from build123d import *

# Parameters (mm, degrees)
EXTRUDE_1_DEPTH          = 35
CUT_EXTRUDE_1_DEPTH      = 30
SKETCH_3_R               = 10
CUT_EXTRUDE_2_DEPTH      = 1
CUT_EXTRUDE_2_DEPTH_BACK = 71
CUT_EXTRUDE_3_DEPTH      = 5
HOLE_WIZARD_M4_1_D       = 3.3
HOLE_WIZARD_M4_1_DEPTH   = 5
HOLE_WIZARD_M4_2_D       = 3.3
HOLE_WIZARD_M4_2_DEPTH   = 5


with BuildPart() as part:
    # 스케치1 → 보스-돌출1 (new body)
    with BuildSketch(Plane(origin=(0, 0, 0), x_dir=(1, 0, 0), z_dir=(0, 1, 0))):
        with BuildLine():
            Line((-26, 35), (26, 35))
            ThreePointArc((26, 35), (61, 0), (26, -35))
            Line((26, -35), (-26, -35))
            ThreePointArc((-26, -35), (-61, 0), (-26, 35))
        make_face()
    extrude(amount=EXTRUDE_1_DEPTH)

    # 스케치2 → 컷-돌출1 (cut)
    with BuildSketch(Plane(origin=(0, 35, 0), x_dir=(1, 0, 0), z_dir=(0, 1, 0))):
        with BuildLine():
            Line((26, 30), (-26, 30))
            ThreePointArc((-26, 30), (-56, 0), (-26, -30))
            Line((-26, -30), (26, -30))
            ThreePointArc((26, -30), (56, 0), (26, 30))
        make_face()
    extrude(amount=-CUT_EXTRUDE_1_DEPTH, mode=Mode.SUBTRACT)

    # 스케치3 → 컷-돌출2 (cut, two sides)
    with BuildSketch(Plane.XY.offset(35)) as cut_extrude_2_sk:
        with Locations((0, 35)):
            Circle(SKETCH_3_R)
    extrude(amount=CUT_EXTRUDE_2_DEPTH, mode=Mode.SUBTRACT)
    extrude(cut_extrude_2_sk.sketch, amount=-CUT_EXTRUDE_2_DEPTH_BACK, mode=Mode.SUBTRACT)

    # 스케치4 → 컷-돌출3 (cut)
    with BuildSketch(Plane(origin=(0, 35, 0), x_dir=(1, 0, 0), z_dir=(0, 1, 0))):
        with BuildLine():
            Line((-26, -32), (26, -32))
            ThreePointArc((26, -32), (58, 0), (26, 32))
            Line((26, 32), (-26, 32))
            ThreePointArc((-26, 32), (-58, 0), (-26, -32))
        make_face()
        with BuildLine():
            Line((-26, -30), (26, -30))
            ThreePointArc((26, -30), (56, 0), (26, 30))
            Line((26, 30), (-26, 30))
            ThreePointArc((-26, 30), (-56, 0), (-26, -30))
        make_face(mode=Mode.SUBTRACT)
    extrude(amount=-CUT_EXTRUDE_3_DEPTH, mode=Mode.SUBTRACT)

    # M4 나사 구멍1
    with Locations(Plane.XY.offset(35)):
        with Locations((-10.606601718, 24.393398282), (10.606601718, 24.393398282)):
            Hole(HOLE_WIZARD_M4_1_D / 2, depth=HOLE_WIZARD_M4_1_DEPTH)

    # M4 나사 구멍2
    with Locations(Plane(origin=(0, 0, -35), x_dir=(-1, 0, 0), z_dir=(0, 0, -1))):
        with Locations((-10.606601718, 24.393398282), (10.606601718, 24.393398282)):
            Hole(HOLE_WIZARD_M4_2_D / 2, depth=HOLE_WIZARD_M4_2_DEPTH)


solid = part.part
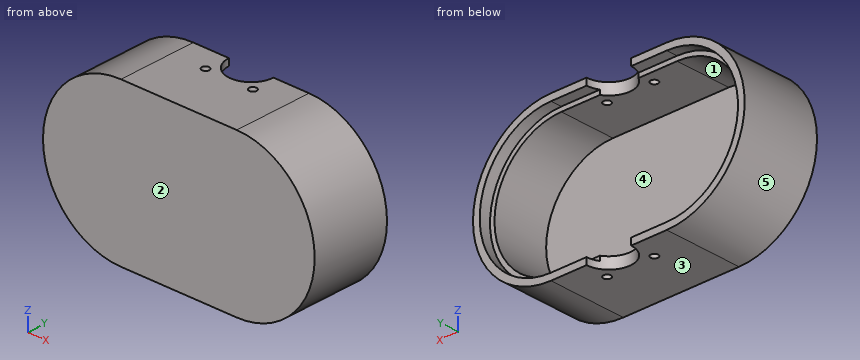
Model file for the job. Use its own axes, mm. Face numbers are marked on the shaded views. A direction names the side the tool comes from. Coordinates: 2 decimals unless noted, no trailing zeros. Write each loop counter-clockwise with the first axis right and the second up, starting at its lowest first coordinate (ties: lowest second). Pieces come first, ordered by that corner, then holes. Notation, with made-up numbers: (5, 44.25) - (53, 44.25) arc R10 ccw to (53, 54.25) - close; hole circle Ø11 at (-17.5, 65.25). An arc over 180 degrees is marked (long way). Write each question's results on one line, items separated by ' | '. Start each with the question number.
1) 3-axis set-ups, long thin cutter, end or side, ignore diameter. For the marked faces 4 and 5: which of +Z, -Z, +X, -X, +Y, -Y reach the whole face in a straight line?
2) Mould opens along Z. For the marked faces 1, 2 and 3 say: pulls with the +Z half, pulls with the -Z half, needs draft (parallel to the pull), parting line crosses it, or undercut.
3) Flat gauge pins, fed straight in: P1, Ø24.5, axis at x = 25.5, z = -7.5, coming from the +Y side; P2, Ø2, axis at y = 9.5, z = 20, coming from the +X side; P3, Ø5.5, axis at x = -10.61, y = 24.39, coming from the -Z side; P4, Ø1, axis at y = 28, z = 8, coming from the +X side. Where does each tip first touch, or does it go through?
4) Cut at A-A (y = 21.5). Write the cut outline in (x, z).
5) Cut at D-D (x = 15.5). Write the cut outline in (y, z).
6) Cut at B-B (x = 0). Write the cut outline in (y, z), then the cut area to 3 significant figures.
7) Probe line 1 along Z through (x, y) = (25, 9); line 2 along Y through (x, z) = (-15.5, 19); line 3 along X through (y, z) = (13.5, -15.5). List the from-to ranges inside material, lowest first. Write a range as from..to.
8) Cut at C-C (z = 0). Write the cut outline in (x, y), then the cut area to 3 significant figures.
Returned:
1) face 4: +Y | face 5: -X, +Y, -Y
2) face 1: undercut | face 2: needs draft | face 3: pulls with the -Z half
3) P1: y = 5 | P2: x = 55.39 | P3: z = -35 | P4: x = 60.19
4) outline: (-26, -35) - (26, -35) arc R35 ccw to (26, 35) - (-26, 35) arc R35 ccw to start; hole (-26, -30) - (26, -30) arc R30 ccw to (26, 30) - (-26, 30) arc R30 ccw to start
5) outline: (0, -35) - (35, -35) - (35, -32) - (30, -32) - (30, -30) - (5, -30) - (5, 30) - (30, 30) - (30, 32) - (35, 32) - (35, 35) - (0, 35) - close
6) outline: (0, -35) - (25, -35) - (25, -30) - (5, -30) - (5, 30) - (25, 30) - (25, 35) - (0, 35) - close | area: 550 mm^2
7) line 1: -35..-30, 30..35 | line 2: 0..5 | line 3: -57.38..-51.69, 51.69..57.38
8) outline: (-61, 0) - (61, 0) - (61, 35) - (58, 35) - (58, 30) - (56, 30) - (56, 5) - (-56, 5) - (-56, 30) - (-58, 30) - (-58, 35) - (-61, 35) - close | area: 890 mm^2
